For this review, use the dimensioned drawing (mm, ordinates from the lowest corner) and the shaded views. Coordinates: 2 decimals unless noted, no trailing zeros. Loops run counter-clockwise (first coordinate to the right, second up) from the corner with the lowest first, then second, coordinate; pieces in that order, holes last. Notation, with made-up numbers: (50, 69) - (71, 69) arc R22 ccw to (71, 106) - close; hole circle Ø7 at (88, 44). An arc over 180 degrees is marked (long way). One line per item, written item: value. Start each with the question number.
1. Insertion check: P1, Ø2, axis at x = 20, z = 9.5, coming from the -Y side; P2, Ø1, axis at x = 56, y = 1.5, coming from the +Z side; P3, Ø0.8, axis at y = 1.5, z = 5.5, coming from the +X side. Each pin has a flat end and moves straight along its axis. Give the tip position at first contact, or say it passes through.
2. To check wall thickness, follow line 1 (X direction, y = 0.9, z = 16.5); line 2 (X direction, y = 1.9, z = 37.5); line 3 (X direction, y = 2.4, z = 12.5). State the ranges of each line that lie inside material, in increasing order.
3. We need section A-A, the plane z = 37.5. Give the boundary of the cut face in (x, y), then the cut area to 3 significant figures.
4. We need section C-C, the plane x = 65. Give the boundary of the cut face in (y, z), then the cut area to 3 significant figures.
5. We need section D-D, the plane z = 20. Give the boundary of the cut face in (x, y), then the cut area to 4 significant figures.
6. We need section B-B, the plane y = 1. Count the separate pieces of the cut face and the enclosed holes in it, then the cut area to 3 significant figures.
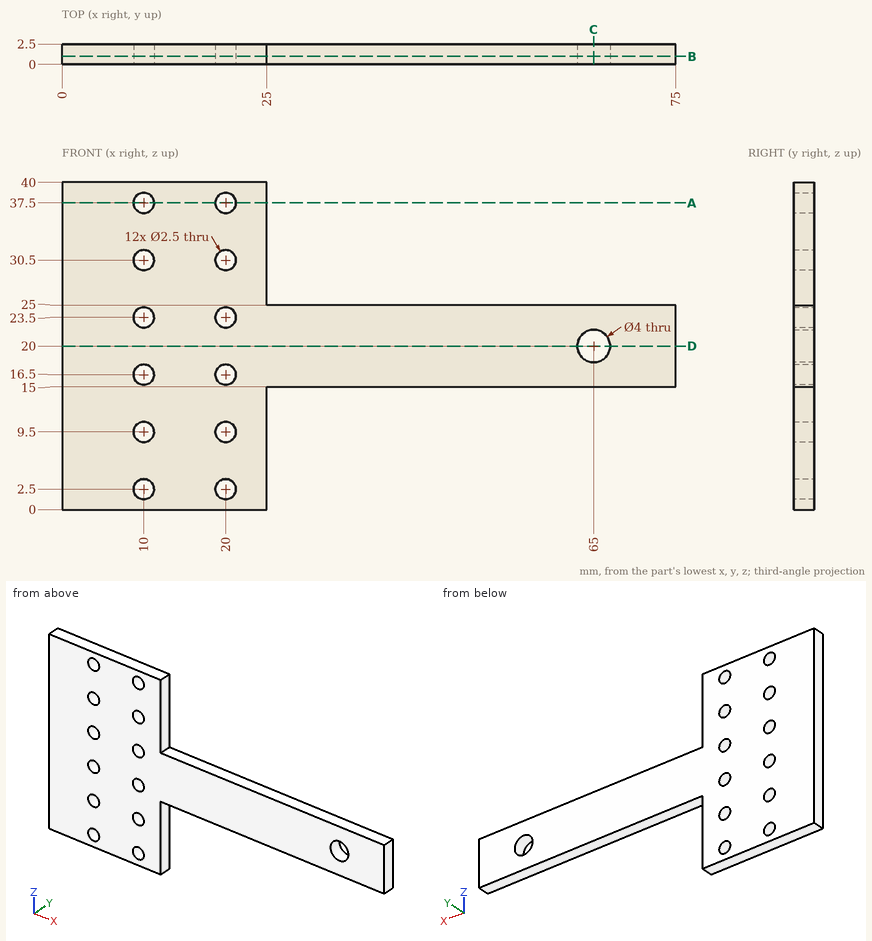
Findings below:
1. P1: through
1. P2: z = 25
1. P3: x = 25
2. line 1: 0 to 8.75, 11.25 to 18.75, 21.25 to 75
2. line 2: 0 to 8.75, 11.25 to 18.75, 21.25 to 25
2. line 3: 0 to 25
3. outline: (0, 0) - (8.75, 0) - (8.75, 2.5) - (0, 2.5) - close; (11.25, 0) - (18.75, 0) - (18.75, 2.5) - (11.25, 2.5) - close; (21.25, 0) - (25, 0) - (25, 2.5) - (21.25, 2.5) - close
3. area: 50.0 mm2
4. outline: (0, 15) - (2.5, 15) - (2.5, 18) - (0, 18) - close; (0, 22) - (2.5, 22) - (2.5, 25) - (0, 25) - close
4. area: 15.0 mm2
5. outline: (0, 0) - (63, 0) - (63, 2.5) - (0, 2.5) - close; (67, 0) - (75, 0) - (75, 2.5) - (67, 2.5) - close
5. area: 177.5 mm2
6. separate pieces: 1
6. enclosed holes: 13
6. area: 1,430 mm2
